Autodesk Fusion 360 part; units mm, degrees
sketch "Sketch1" plane through (0, 0, 0) normal (0, 0, 1) x (1, 0, 0)
  line L0 (0, 0) -> (10, 0)
  line L1 (10, 0) -> (10, 10)
  line L2 (10, 10) -> (0, 10)
  line L3 (0, 10) -> (0, 0)
  dimension "d1" = 10
  dimension "d2" = 10
extrude "Extrude1" add sketch "Sketch1" along normal blind 25
sketch "Sketch2" plane through (0, 0, 0) normal (0, -1, 0) x (1, 0, 0)
  line L0 (0, 0) -> (10, 0)
  line L1 (10, 0) -> (10, 25)
  line L2 (10, 25) -> (0, 25)
  line L3 (0, 25) -> (0, 0)
  circle A0 centre (5, 20) radius 4
  dimension "d5" = 8
extrude "Extrude2" cut sketch "Sketch2" against normal blind 10 contours A0
sketch "Sketch3" plane through (0, 0, 0) normal (0, 0, -1) x (1, 0, 0)
  line L0 (0, 0) -> (0, -10)
  line L1 (0, -10) -> (10, -10)
  line L2 (10, -10) -> (10, 0)
  line L3 (10, 0) -> (0, 0)
  circle A0 centre (5, -5) radius 3.75
  dimension "d8" = 7.5
extrude "Extrude3" add sketch "Sketch3" along normal blind 10 contours A0
Geometry check sheet. Reference: the model listing, model coordinates, mm. A direction names the side the tool comes from. Give positions to 0.01 mm unless a question says otherwise; leave off trailing zeros. Order: outer loops, then holes, each group sorted by start corner. A loop starts at its lowest first (then second) coordinate and runs counter-clockwise, first axis right, second up.
1. Sectioned sample at A-A (z = 20). Record the boundary of the cut face in (x, y), then the cut area to 3 significant figures.
Completed:
outline: (0, 0) - (1, 0) - (1, 10) - (0, 10) - close; (9, 0) - (10, 0) - (10, 10) - (9, 10) - close
area: 20.0 mm2
2. Scan lines: line 1 (Z direction, x = 5, y = 6.5); line 2 (Z direction, x = 9.25, y = 1.25); line 3 (X direction, y = 2.5, z = 21). Record each from-to range of solid material in increasing order.
Completed:
line 1: z = -10 to 16, 24 to 25
line 2: z = 0 to 25
line 3: x = 0 to 1.13, 8.87 to 10
3. Access from +Z, -Z, +X, -X, +Y, -Y to the whole of each face (thin tool, end or side, straight path). Record for faces 1 (the face through (2.7, 8.4, 0)), 2 (the face through (10, 5, 12)).
Completed:
face 1: -Z
face 2: +Z, -Z, +X, +Y, -Y
4. Sectioned sample at C-C (y = 5). Record the boundary of the cut face in (x, z).
Completed:
outline: (0, 0) - (1.25, 0) - (1.25, -10) - (8.75, -10) - (8.75, 0) - (10, 0) - (10, 25) - (0, 25) - close; hole circle Ø8 at (5, 20)
5. Sectioned sample at D-D (x = 7). Record the boundary of the cut face in (y, z).
Completed:
outline: (0, 0) - (1.83, 0) - (1.83, -10) - (8.17, -10) - (8.17, 0) - (10, 0) - (10, 16.54) - (0, 16.54) - close; (0, 23.46) - (10, 23.46) - (10, 25) - (0, 25) - close
6. Depth check by flat-ended pin: pin 1 (5 mm diameter, centred on x = 5, z = 20, fed in from -Y); pin 2 (4 mm diameter, centred on x = 2.5, z = 11, fed in from -Y). Enter the tip coordinate at first touch or a pass-through.
Completed:
pin 1: passes through
pin 2: stops at y = 0
7. Sectioned sample at B-B (x = 5). Record the boundary of the cut face in (y, z), then the cut area to 3 significant figures.
Completed:
outline: (0, 0) - (1.25, 0) - (1.25, -10) - (8.75, -10) - (8.75, 0) - (10, 0) - (10, 16) - (0, 16) - close; (0, 24) - (10, 24) - (10, 25) - (0, 25) - close
area: 245 mm2
8. Draft check along Z on faces 3 (the face through (4.479, 4.93, 23.966)), 4 (the face through (5, 5, 25)), 5 (the face through (0, 5, 12)), 6 (the face through (5, 5, -10)). Enter one of: pulls with the +Z half, pulls with the -Z half, needs draft (parallel to the pull), parting line crosses it, or undercut.
Completed:
face 3: undercut
face 4: pulls with the +Z half
face 5: needs draft
face 6: pulls with the -Z half
